Geometry: final body of the model. Coordinates: model frame, mm. Give positions to 0.01 mm unless a question says otherwise; leave off trailing zeros. Write each loop counter-clockwise with the first axis right and the second up, starting at its lowest first coordinate (ties: lowest second). Pieces come first, ordered by that corner, then holes. Notation, with made-up numbers: (79, 43.25) - (110, 43.25) arc R21 ccw to (110, 52.25) - close; hole circle Ø5 at (13.25, -22.5). An arc over 180 degrees is marked (long way). Use CSV: the item, a comma, the result in double quotes. Start each with the question number.
(1) First-contact query: pin 1 Ø2.5 at (x, z) = (43, -29) entering from -Y. Flat tip, straight axial feed; report the tip coordinate or a pass-through.
(2) Section D-D on z = -17.5. Output: boundary loops of the cut face in (x, y), and give its area (3 significant figures).
(3) Line query: probe 1 along X at (y, z) = (0.6, 21.5); probe 2 along X at (y, z) = (1.6, -29); probe 3 along X at (y, z) = (1.3, 29). Output: solid intervals per line, ascending. Write a range as [from, to].
(4) Section A-A on x = 26.5. Output: boundary loops of the cut face in (y, z).
(5) Section B-B on z = 21.5. Output: boundary loops of the cut face in (x, y).
(6) Section C-C on z = 36.5. Output: boundary loops of the cut face in (x, y).
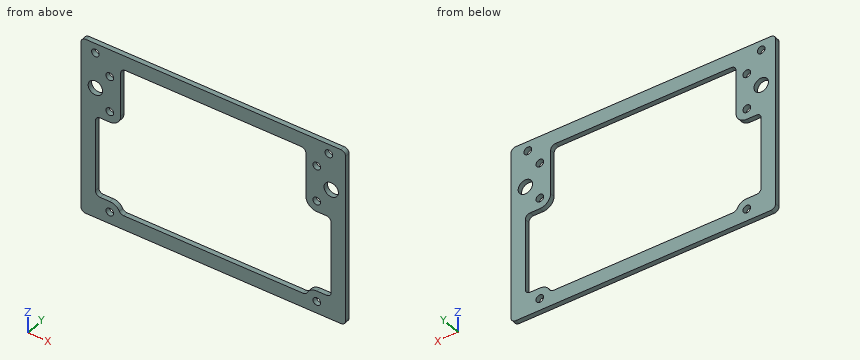
from build123d import *

# Parameters (mm, degrees)
SKETCH_1_W          = 110
SKETCH_1_H          = 79
SKETCH_1_R          = 1.6
EXTRUDE_1_DEPTH     = 2
SKETCH_3_W          = 110
SKETCH_3_H          = 1
EXTRUDE_2_DEPTH     = 2
SKETCH_4_R          = 1.6
CUT_EXTRUDE_2_DEPTH = 2
SKETCH_6_W          = 110
SKETCH_6_H          = 5.5
CUT_EXTRUDE_4_DEPTH = 2
SKETCH_7_R          = 3
CUT_EXTRUDE_5_DEPTH = 2
FILLET_2_R          = 2


with BuildPart() as part:
    # 草图1 → 凸台-拉伸1 (new body)
    with BuildSketch(Plane(origin=(0, 0, 0), x_dir=(1, 0, 0), z_dir=(0, 1, 0))):
        Rectangle(SKETCH_1_W, SKETCH_1_H)
        with Locations(Location((43, -29, 0), (0, 0, 270))):
            Circle(SKETCH_1_R, mode=Mode.SUBTRACT)
        with Locations(Location((-43, -29, 0), (0, 0, 270))):
            Circle(SKETCH_1_R, mode=Mode.SUBTRACT)
        with Locations(Location((-43, 29, 0), (0, 0, 270))):
            Circle(SKETCH_1_R, mode=Mode.SUBTRACT)
        with Locations(Location((43, 29, 0), (0, 0, 270))):
            Circle(SKETCH_1_R, mode=Mode.SUBTRACT)
        with Locations(Location((43, -14, 0), (0, 0, 270))):
            Circle(SKETCH_1_R, mode=Mode.SUBTRACT)
        with Locations(Location((-43, -14, 0), (0, 0, 270))):
            Circle(SKETCH_1_R, mode=Mode.SUBTRACT)
    extrude(amount=EXTRUDE_1_DEPTH)

    # 草图3 → 凸台-拉伸2 (add)
    with BuildSketch(Plane(origin=(0, 2, 0), x_dir=(1, 0, 0), z_dir=(0, 1, 0))):
        with Locations((0, -40)):
            Rectangle(SKETCH_3_W, SKETCH_3_H)
    extrude(amount=-EXTRUDE_2_DEPTH)

    # 草图4 → 切除-拉伸2 (cut)
    with BuildSketch(Plane(origin=(0, 2, 0), x_dir=(1, 0, 0), z_dir=(0, 1, 0))):
        with Locations(Location((48, -36.5, 0), (0, 0, 270))):
            Circle(SKETCH_4_R)
        with Locations(Location((-49, -36.5, 0), (0, 0, 270))):
            Circle(SKETCH_4_R)
    extrude(amount=-CUT_EXTRUDE_2_DEPTH, mode=Mode.SUBTRACT)

    # 草图6 → 切除-拉伸4 (cut)
    with BuildSketch(Plane(origin=(0, 2, 0), x_dir=(1, 0, 0), z_dir=(0, 1, 0))):
        with Locations((0, 36.75)):
            Rectangle(SKETCH_6_W, SKETCH_6_H)
        with BuildLine():
            Line((-38.612517806, 28), (38.612517806, 28))
            ThreePointArc((38.612517806, 28), (40.19375696, 25.48218818), (43, 24.5))
            Line((43, 24.5), (49, 24.5))
            Line((49, 24.5), (49, -9.5))
            Line((49, -9.5), (43, -9.5))
            ThreePointArc((43, -9.5), (39.818019485, -10.818019485), (38.5, -14))
            Line((38.5, -14), (38.5, -34.5))
            Line((38.5, -34.5), (-38.5, -34.5))
            Line((-38.5, -34.5), (-38.5, -14))
            ThreePointArc((-38.5, -14), (-39.818019485, -10.818019485), (-43, -9.5))
            Line((-43, -9.5), (-49, -9.5))
            Line((-49, -9.5), (-49, 24.5))
            Line((-49, 24.5), (-43, 24.5))
            ThreePointArc((-43, 24.5), (-40.19375696, 25.48218818), (-38.612517806, 28))
        make_face()
    extrude(amount=-CUT_EXTRUDE_4_DEPTH, mode=Mode.SUBTRACT)

    # 草图7 → 切除-拉伸5 (cut)
    with BuildSketch(Plane(origin=(0, 2, 0), x_dir=(1, 0, 0), z_dir=(0, 1, 0))):
        with Locations(Location((49, -21.5, 0), (0, 0, 270))):
            Circle(SKETCH_7_R)
        with Locations(Location((-49, -21.5, 0), (0, 0, 90))):
            Circle(SKETCH_7_R)
    extrude(amount=-CUT_EXTRUDE_5_DEPTH, mode=Mode.SUBTRACT)

    # 圆角2
    fillet_2_edges = [part.edges().sort_by_distance(p)[0] for p in [
        (-55, 1, 40.5),
        (55, 1, 40.5),
        (38.5, 1, 34.5),
        (-38.5, 1, 34.5),
        (-49, 1, 9.5),
        (-49, 1, -24.5),
        (-38.612517806, 1, -28),
        (38.612517806, 1, -28),
        (49, 1, -24.5),
        (49, 1, 9.5),
        (-55, 1, -34),
        (55, 1, -34),
    ]]
    fillet(fillet_2_edges, radius=FILLET_2_R)


solid = part.part
Check values:
1,pin 1,"passes through"
2,outline,"(-55, 0) - (-49, 0) - (-49, 2) - (-55, 2) - close; (49, 0) - (55, 0) - (55, 2) - (49, 2) - close"
2,area,"24.0 mm²"
3,probe 1,"x = [-55, -52], [-46, -38.5], [38.5, 46], [52, 55]"
3,probe 2,"x = [-55, -44.6], [-41.4, 41.4], [44.6, 55]"
3,probe 3,"x = [-55, -44.6], [-41.4, -38.5], [38.5, 41.4], [44.6, 55]"
4,outline,"(0, -34) - (2, -34) - (2, -28) - (0, -28) - close; (0, 34.5) - (2, 34.5) - (2, 40.5) - (0, 40.5) - close"
5,outline,"(-55, 0) - (-52, 0) - (-52, 2) - (-55, 2) - close; (-46, 0) - (-38.5, 0) - (-38.5, 2) - (-46, 2) - close; (38.5, 0) - (46, 0) - (46, 2) - (38.5, 2) - close; (52, 0) - (55, 0) - (55, 2) - (52, 2) - close"
6,outline,"(-55, 0) - (-50.6, 0) - (-50.6, 2) - (-55, 2) - close; (-47.4, 0) - (46.4, 0) - (46.4, 2) - (-47.4, 2) - close; (49.6, 0) - (55, 0) - (55, 2) - (49.6, 2) - close"
